```python
from build123d import *

# Parameters (mm, degrees)
F0_W     = 60
F0_H     = 20
F0_W_2   = 54
F0_H_2   = 14
F1_DEPTH = 3.5
F2_R     = 3


with BuildPart() as f1:
    # F0 (on Top) → F1 (new body, symmetric)
    with BuildSketch(Plane.XY):
        Rectangle(F0_W, F0_H)
        Rectangle(F0_W_2, F0_H_2, mode=Mode.SUBTRACT)
    extrude(amount=F1_DEPTH, both=True)

    # F2
    f2_edges = [f1.edges().sort_by_distance(p)[0] for p in [
        (-30, -10, 0),
        (-30, 10, 0),
        (-27, 7, 0),
        (-27, -7, 0),
        (27, 7, 0),
        (27, -7, 0),
        (30, 10, 0),
        (30, -10, 0),
    ]]
    fillet(f2_edges, radius=F2_R)


solid = f1.part
```
Source: CAD feature listing. Evaluate the final solid. Frame: model axes, mm. A direction names the side the tool comes from. Coordinates: 2 decimals unless noted, no trailing zeros. Order: outer loops, then holes, each group sorted by start corner. A loop starts at its lowest first (then second) coordinate and runs counter-clockwise, first axis right, second up. Notation, with made-up numbers: M 12,9.25 L 26,9.25 A19 ccw 26,35.25 Z; hole C -20.75,77 d1. An arc over 180 degrees is marked long. Write each question's results on one line, items separated by ' | '. Start each with the question number.
1) Access query for faces 5 (the face through (-26.14, 6.1, -0.05)), 6 (the face through (-29.14, -9.1, 0.05)). Directions: +Z, -Z, +X, -X, +Y, -Y. A direction counts if a zero-diameter tool reaches every point of the face in a straight line with its end or side. Return the directions, or none.
2) Section query B-B (x = 9.5). Return the cut outline in (y, z), plus the area to 3 significant figures.
3) Line query: line 1 (Y direction, x = -13, z = -1.75); line 2 (X direction, y = 2.25, z = -1.25); line 3 (X direction, y = -5.75, z = 0). Output: solid intervals per line, ascending. Write a range as from..to.
4) Draft query along X for faces 1 (the face through (29.14, -9.1, 0.05)), 2 (the face through (-26.14, -6.1, 0.05)), 3 (the face through (-29.14, 9.1, -0.05)), 4 (the face through (-27, 0, 0)). Return one class per face: released by +X, released by -X, zero draft, split by the parting line, or undercut.
5) Section query A-A (z = 2.25). Return the cut outline in (x, y).
6) Section query C-C (y = 3). Return the cut outline in (x, z), plus the area to 3 significant figures.
Answers:
1) face 5: +Z, -Z | face 6: +Z, -Z, -X, -Y
2) outline: M -10,-3.5 L -7,-3.5 L -7,3.5 L -10,3.5 Z; M 7,-3.5 L 10,-3.5 L 10,3.5 L 7,3.5 Z | area: 42.0 mm^2
3) line 1: y = -10..-7, 7..10 | line 2: x = -30..-27, 27..30 | line 3: x = -30..-26.44, 26.44..30
4) face 1: released by +X | face 2: undercut | face 3: released by -X | face 4: undercut
5) outline: M -30,-7 A3 ccw -27,-10 L 27,-10 A3 ccw 30,-7 L 30,7 A3 ccw 27,10 L -27,10 A3 ccw -30,7 Z; hole M -27,-4 A3 ccw -24,-7 L 24,-7 A3 ccw 27,-4 L 27,4 A3 ccw 24,7 L -24,7 A3 ccw -27,4 Z
6) outline: M -30,-3.5 L -27,-3.5 L -27,3.5 L -30,3.5 Z; M 27,-3.5 L 30,-3.5 L 30,3.5 L 27,3.5 Z | area: 42.0 mm^2
